Autodesk Inventor part; units mm, degrees
ref_plane "YZ Plane" through (0, 0, 0) normal (1, 0, 0) x (0, 1, 0)
ref_plane "XZ Plane" through (0, 0, 0) normal (0, 1, 0) x (-1, 0, 0)
ref_plane "XY Plane" through (0, 0, 0) normal (0, 0, 1) x (1, 0, 0)
sketch "Sketch1" plane through (0, 0, 0) normal (0, 0, 1) x (1, 0, 0)
  circle A0 centre (0, 0) radius 18.5
  circle A1 centre (0, 0) radius 19.5
  line L0 (0, 0) -> (0, 25.1943)
  arc A2 (5, 23) -> (-5, 23) centre (0, 23) ccw
  line L1 (5, 23) -> (5, 18.8481)
  line L2 (-5, 23) -> (-5, 18.8481)
  circle A3 centre (0, 23) radius 2.5
  point P0 (-5, 25.1943)
  point P1 (5, 25.1943)
  dimension "d0" = 37
  dimension "d1" = 1
  dimension "d16" = 10
  dimension "d17" = 23
  dimension "d18" = 5
extrude "Extrusion1" add sketch "Sketch1" against normal blind 1 contours A0 | A1
extrude "Extrusion2" add sketch "Sketch1" along normal blind 36 contours A1
sketch "Sketch2" plane through (0, 0, 0) normal (1, 0, 0) x (0, 1, 0)
  line L0 (19.5, 36) -> (-19.5, 36)
  line L1 (12, 36) -> (-19.5, 12)
  line L2 (-19.5, 36) -> (-19.5, -1)
  line L3 (12, 36) -> (19.5, 36)
  line L4 (-19.5, 12) -> (-19.5, -1)
  line L5 (-19.5, -1) -> (19.5, -1)
  line L6 (-19.5, -1) -> (19.5, -1)
  line L7 (19.5, -1) -> (19.5, 36)
  point P0 (0, 0)
  dimension "d7" = 12
  dimension "d8" = 12
extrude "Extrusion3" cut sketch "Sketch2" along normal mid plane 50 contours L1 L2 L0
sketch "Sketch3" plane through (0, 0, 0) normal (0, 1, 0) x (-1, 0, 0)
  line L0 (18.5, 0) -> (-18.5, 0)
  line L1 (5, 0) -> (-5, 0)
  line L2 (-5, 0) -> (-5, 14)
  line L3 (-5, 14) -> (5, 14)
  line L4 (5, 14) -> (5, 0)
  point P0 (0, 0)
  dimension "d11" = 5
  dimension "d12" = 10
  dimension "d13" = 14
extrude "Extrusion4" cut sketch "Sketch3" along normal mid plane 50
extrude "Extrusion5" add sketch "Sketch1" against normal blind 1 contours A1 L2 A2 L1
properties part number "CatWaterSensorCase"
Source: CAD feature listing. Evaluate the final solid. Frame: model axes, mm. A direction names the side the tool comes from. Give positions to 0.01 mm unless a question says otherwise; leave off trailing zeros. Loops run counter-clockwise (first coordinate to the right, second up) from the corner with the lowest first, then second, coordinate; pieces in that order, holes last. Notation, with made-up numbers: (58, 10.5) - (62, 10.5) arc R28 cw to (62, 46.5) - close; hole circle Ø2 at (33, 57.5). An arc over 180 degrees is marked (long way). Use CSV: the item, a comma, the result in double quotes. Start each with the question number.
1. Reachability of faces 1 (the flat face through (-18.191, -4.495, 23.433)), 2 (the flat face through (0, 19, 14)) from +Z, -Z, +X, -X, +Y, -Y: full face, straight path, thin tool, end or side. Return the list, or none.
2. Section A-A (x = 0). Output: boundary loops of the cut face in (y, z).
3. Section B-B (z = 11). Output: boundary loops of the cut face in (x, y).
4. Draft query along X for faces 3 (the flat face through (1, 19, 36)), 4 (the cylindrical face through (0.1, 28, -0.5)), 5 (the cylindrical face through (-0.743, 18.485, 17.748)), 6 (the flat face through (0, -1, 0)). Return one class per face: +X half, -X half, draft (parallel to the pull), parting line (faces both ways), or undercut.
5. Ray query, L1, parallel to Y at x = 0, z = -0.15; L2, parallel to X at y = 0, z = 20; L3, parallel to X at y = 23, z = -0.45. Return the intervals inside material, ascending.
6. Pin query (flat end, axial travel): pin 1 (1 mm diameter, centred on y = 0.5, z = 19, fed in from +X); pin 2 (6.5 mm diameter, centred on x = 0, y = 23, fed in from +Z); pin 3 (0.5 mm diameter, centred on y = 20.5, z = -0.5, fed in from +X); pin 4 (1.5 mm diameter, centred on y = 13, z = 6.5, fed in from -X). Return the tip coordinate at first contact, or that it passes through.
7. Section C-C (y = 24). Output: boundary loops of the cut face in (x, z), then the cut area to 3 significant figures.
8. Section D-D (x = -8). Output: boundary loops of the cut face in (y, z), then the cut area to 3 significant figures.
Response:
1,face 1,"+Z, +X, -X, -Y"
1,face 2,"+Y, -Y"
2,outline,"(-19.5, -1) - (20.5, -1) - (20.5, 0) - (-19.5, 0) - close; (18.5, 14) - (19.5, 14) - (19.5, 36) - (18.5, 36) - close; (25.5, -1) - (28, -1) - (28, 0) - (25.5, 0) - close"
3,outline,"(-5, -18.85) - (-5, -17.81) arc R18.5 cw to (-5, 17.81) - (-5, 18.85) arc R19.5 ccw to start; (5, -18.85) arc R19.5 ccw to (5, 18.85) - (5, 17.81) arc R18.5 cw to (5, -17.81) - close"
4,face 3,"draft"
4,face 4,"parting line"
4,face 5,"undercut"
4,face 6,"undercut"
5,L1,"-19.5 to 20.5, 25.5 to 28"
5,L2,"-19.5 to -18.5, 18.5 to 19.5"
5,L3,"-5 to -2.5, 2.5 to 5"
6,pin 1,"x = 19.5"
6,pin 2,"z = 0"
6,pin 3,"x = 5"
6,pin 4,"x = -15.17"
7,outline,"(-4.9, -1) - (-2.29, -1) - (-2.29, 0) - (-4.9, 0) - close; (2.29, -1) - (4.9, -1) - (4.9, 0) - (2.29, 0) - close"
7,area,"5.22 mm²"
8,outline,"(-17.78, -1) - (17.78, -1) - (17.78, 36) - (16.68, 36) - (16.68, 0) - (-16.68, 0) - (-16.68, 14.15) - (-17.78, 13.31) - close"
8,area,"90.4 mm²"
